from build123d import *

# Parameters (mm, degrees)
PAD_DEPTH       = 50
SKETCH001_R     = 11
SKETCH001_R_2   = 2
POCKET_DEPTH    = 3
POCKET001_DEPTH = 3
CHAMFER_SIZE    = 5
FILLET_R        = 2
PAD001_DEPTH    = 2
PAD002_DEPTH    = 2


with BuildPart() as part:
    # Sketch → Pad (new body)
    with BuildSketch(Plane.XY):
        Polygon((-28, 24), (-25, 24), (-25, -24), (25, -24), (25, -27), (-28, -27), align=None)
    extrude(amount=PAD_DEPTH)

    # Sketch001 (on Face2 of Pad) → Pocket (cut)
    with BuildSketch(Plane.YZ.offset(-25)):
        with Locations((3, 25)):
            Circle(SKETCH001_R)
        with Locations((-12.5, 40.5)):
            Circle(SKETCH001_R_2)
        with Locations((18.5, 40.5)):
            Circle(SKETCH001_R_2)
        with Locations((-12.5, 9.5)):
            Circle(SKETCH001_R_2)
        with Locations((18.5, 9.5)):
            Circle(SKETCH001_R_2)
    extrude(amount=-POCKET_DEPTH, mode=Mode.SUBTRACT)

    # Sketch002 (on Face12 of Pocket) → Pocket001 (cut)
    with BuildSketch(Plane(origin=(0, -24, 0), x_dir=(-1, 0, 0), z_dir=(0, 1, 0))):
        with BuildLine():
            ThreePointArc((-14, 42.15), (-16.15, 40), (-14, 37.85))
            Line((-14, 37.85), (16, 37.85))
            ThreePointArc((16, 37.85), (18.15, 40), (16, 42.15))
            Line((-14, 42.15), (16, 42.15))
        make_face()
        with BuildLine():
            ThreePointArc((-14, 12.15), (-16.15, 10), (-14, 7.85))
            Line((-14, 7.85), (16, 7.85))
            ThreePointArc((16, 7.85), (18.15, 10), (16, 12.15))
            Line((-14, 12.15), (16, 12.15))
        make_face()
    extrude(amount=-POCKET001_DEPTH, mode=Mode.SUBTRACT)

    # Chamfer
    chamfer_edges = [part.edges().sort_by_distance(p)[0] for p in [
        (-26.5, 24, 0),
        (25, -25.5, 0),
        (-26.5, 24, 50),
        (25, -25.5, 50),
    ]]
    chamfer(chamfer_edges, length=CHAMFER_SIZE)

    # Fillet
    fillet_edges = [part.edges().sort_by_distance(p)[0] for p in [
        (-28, -27, 25),
    ]]
    fillet(fillet_edges, radius=FILLET_R)

    # Sketch003 (on Face5 of Fillet) → Pad001 (join)
    with BuildSketch(Plane.XY.offset(50)):
        Polygon((-25, -24), (-12, -24), (-25, -4), align=None)
    extrude(amount=-PAD001_DEPTH)

    # Sketch004 (on Face2 of Pad001) → Pad002 (join)
    with BuildSketch(Plane(origin=(0, 0, 0), x_dir=(1, 0, 0), z_dir=(0, 0, -1))):
        Polygon((-25, 24), (-12, 24), (-25, 4), align=None)
    extrude(amount=-PAD002_DEPTH)


solid = part.part
Source: CAD feature listing. Evaluate the final solid. Frame: model axes, mm. A direction names the side the tool comes from. Round coordinates to 2 decimals unless told otherwise and drop trailing zeros. Loops run counter-clockwise (first coordinate to the right, second up) from the corner with the lowest first, then second, coordinate; pieces in that order, holes last. Notation, with made-up numbers: (-24, 75.5) -> (28, 75.5) arc R18 cw to (28, 81.5) -> close; hole circle Ø1 at (-40, 56.5). An arc over 180 degrees is marked (long way). Answer as a JSON object with one key per item and string values. Group by question number.
Q1. Section query D-D (y = -1.5). Output: boundary loops of the cut face in (x, z).
Q2. Ray query, line 1 (Z direction, x = -26.4, y = 18.5); line 2 (Z direction, x = -21, y = -15.5); line 3 (Y direction, x = -27, z = 9). Return the intervals inside material, ascending. Write a range as from..to.
Q3. Mould query, pull axis Y, two halves, no side actions, for faces 4 (the flat face through (0, -27, 25)), 5 (the cylindrical face through (16.15, -25.48, 40.05)), 6 (the cylindrical face through (-26.479, 17.026, 10.852)). Classes: pulls with the +Y half, pulls with the -Y half, needs draft (parallel to the pull), parting line crosses it, or undercut.
Q4. Section query C-C (y = -23). Output: boundary loops of the cut face in (x, z), plus the area to 3 significant figures.
Q5. Section query B-B (x = -4). Output: boundary loops of the cut face in (y, z), plus the area to 3 significant figures.
Q6. Section query A-A (z = 25). Output: boundary loops of the cut face in (x, y), plus the area to 3 significant figures.
Q7. Access query for faces 1 (the flat face through (-25, -10, 25)), 2 (the flat face through (-18.41, -14.14, 0.99)), 3 (the cylindrical face through (16.15, -25.48, 10.05)). Directions: +Z, -Z, +X, -X, +Y, -Y. A direction counts if a zero-diameter tool reaches every point of the face in a straight line with its end or side. Return the directions, or none.
Q8. Contact query for flat-ended pins moving along their axis: P1, Ø3, axis at x = -6.5, z = 44, coming from the +Y side; P2, Ø14.5, axis at y = -9.5, z = 23, coming from the +X side. Output: stop coordinate, or through.
Completed:
{
 "1": {"outline": "(-28, 0) -> (-25, 0) -> (-25, 14.96) -> (-28, 14.96) -> close; (-28, 35.04) -> (-25, 35.04) -> (-25, 50) -> (-28, 50) -> close"},
 "2": {"line 1": "0..7.5, 11.5..38.5, 42.5..50", "line 2": "0..2, 48..50", "line 3": "-26.73..-14.44, -10.56..16.56, 20.44..24"},
 "3": {"face 4": "pulls with the -Y half", "face 5": "needs draft", "face 6": "undercut"},
 "4": {"outline": "(-28, 0) -> (-12.65, 0) -> (-12.65, 2) -> (-25, 2) -> (-25, 48) -> (-12.65, 48) -> (-12.65, 50) -> (-28, 50) -> close", "area": "199 mm²"},
 "5": {"outline": "(-27, 0) -> (-24, 0) -> (-24, 7.85) -> (-27, 7.85) -> close; (-27, 12.15) -> (-24, 12.15) -> (-24, 37.85) -> (-27, 37.85) -> close; (-27, 42.15) -> (-24, 42.15) -> (-24, 50) -> (-27, 50) -> close", "area": "124 mm²"},
 "6": {"outline": "(-28, -25) arc R2 ccw to (-26, -27) -> (25, -27) -> (25, -24) -> (-25, -24) -> (-25, -8) -> (-28, -8) -> close; (-28, 14) -> (-25, 14) -> (-25, 24) -> (-28, 24) -> close", "area": "236 mm²"},
 "7": {"face 1": "+X, +Y", "face 2": "+Z, -Z, +X, +Y", "face 3": "+Y, -Y"},
 "8": {"P1": "y = -24", "P2": "x = -25"}
}
